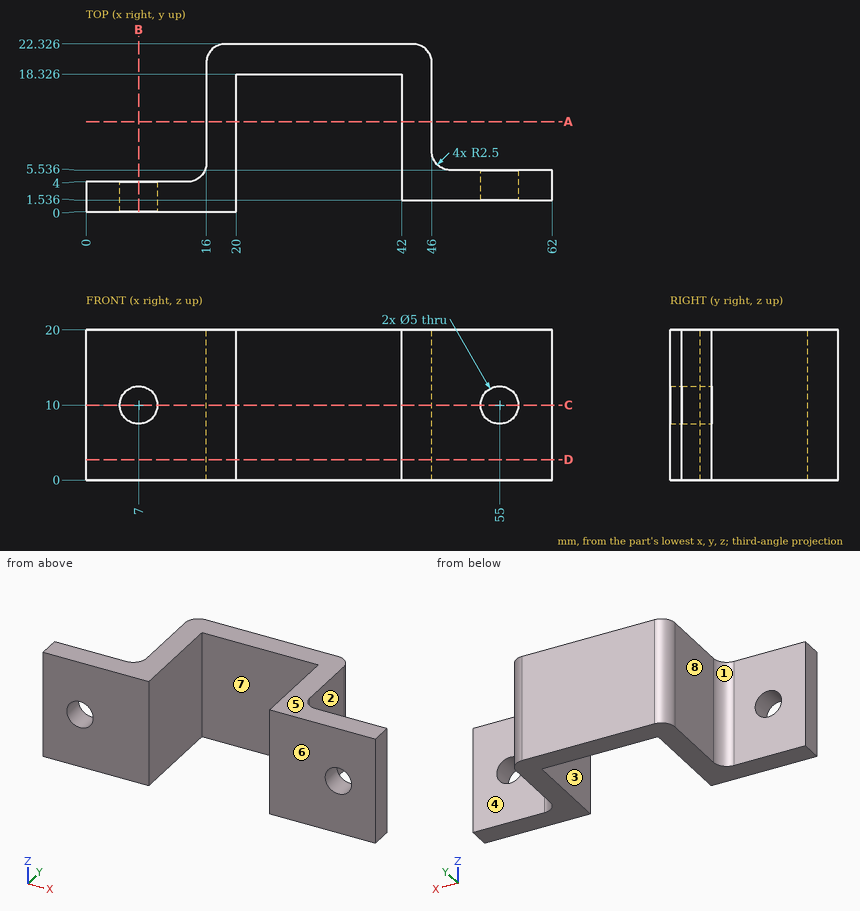
Part print with two shaded views. Sizes in mm from the minimum x, y, z corner. A direction names the side the tool comes from. Coordinates: 2 decimals unless noted, no trailing zeros. Order: outer loops, then holes, each group sorted by start corner. A loop starts at its lowest first (then second) coordinate and runs counter-clockwise, first axis right, second up. Notation, with made-up numbers: M 15,89 L 42,89 A23 ccw 42,101 Z; hole C 4.5,3.5 d2. An arc over 180 degrees is marked long. Use a Markdown table: item, result.
(1) Cut at D-D on z = 2.75. Write the cut outline in (x, y).
A:
| item | result |
|---|---|
| outline | M 0,0 L 20,0 L 20,18.33 L 42,18.33 L 42,1.54 L 62,1.54 L 62,5.54 L 48.5,5.54 A2.5 cw 46,8.04 L 46,19.83 A2.5 ccw 43.5,22.33 L 18.5,22.33 A2.5 ccw 16,19.83 L 16,6.5 A2.5 cw 13.5,4 L 0,4 Z |
(2) Probe L1, parallel to X at y = 2.85, z = 10; L2, parallel to Z at x = 55, y = 4.05; L3, parallel to X at y = 17.5, z = 16.25. List the from-to ranges inside material, lowest first.
A:
| item | result |
|---|---|
| L1 | x = 0 to 4.5, 9.5 to 20, 42 to 52.5, 57.5 to 62 |
| L2 | z = 0 to 7.5, 12.5 to 20 |
| L3 | x = 16 to 20, 42 to 46 |
(3) Tool access for the marked faces 4, 5, 6, 7 and 8: list every direction of +Z, -Z, +X, -X, +Y, -Y with a clear straight run to the whole face (end or side of a thin tool).
A:
| item | result |
|---|---|
| face 4 | +Z, -Z, +X, +Y |
| face 5 | +Z, +X, -X, +Y, -Y |
| face 6 | +Z, -Z, +X, -Y |
| face 7 | +Z, -Z, -Y |
| face 8 | +Z, -Z, -X, +Y |
(4) Cut at C-C on z = 10. Write the cut outline in (x, y).
A:
| item | result |
|---|---|
| outline | M 0,0 L 4.5,0 L 4.5,4 L 0,4 Z; M 9.5,0 L 20,0 L 20,18.33 L 42,18.33 L 42,1.54 L 52.5,1.54 L 52.5,5.54 L 48.5,5.54 A2.5 cw 46,8.04 L 46,19.83 A2.5 ccw 43.5,22.33 L 18.5,22.33 A2.5 ccw 16,19.83 L 16,6.5 A2.5 cw 13.5,4 L 9.5,4 Z; M 57.5,1.54 L 62,1.54 L 62,5.54 L 57.5,5.54 Z |
(5) Cut at A-A on y = 12. Write the cut outline in (x, z), then the cut area to 3 significant figures.
A:
| item | result |
|---|---|
| outline | M 16,0 L 20,0 L 20,20 L 16,20 Z; M 42,0 L 46,0 L 46,20 L 42,20 Z |
| area | 160 mm^2 |
(6) Cut at B-B on x = 7. Write the cut outline in (y, z).
A:
| item | result |
|---|---|
| outline | M 0,0 L 4,0 L 4,7.5 L 0,7.5 Z; M 0,12.5 L 4,12.5 L 4,20 L 0,20 Z |
(7) Pull direction X, two halves, no side cores. Call the marked faces 1, 2 and 3: released by +X, released by -X, zero draft, split by the parting line, or undercut.
A:
| item | result |
|---|---|
| face 1 | released by -X |
| face 2 | released by +X |
| face 3 | undercut |
(8) Flat gauge pins, fed straight in: pin 1 (2 mm diameter, centred on x = 7.5, z = 14.5, fed in from +Y); pin 2 (10.5 mm diameter, centred on y = 10.5, z = 11, fed in from -X) (1 decimal); pin 3 (1.5 mm diameter, centred on y = 12.5, z = 17.5, fed in from +X). Where does each tip first touch, or does it go through?
A:
| item | result |
|---|---|
| pin 1 | stops at y = 4 |
| pin 2 | stops at x = 15.7 |
| pin 3 | stops at x = 46 |
